Part model, mm, in its own coordinate system. A direction names the side the tool comes from. Give positions to 0.01 mm unless a question says otherwise; leave off trailing zeros. Write each loop counter-clockwise with the first axis right and the second up, starting at its lowest first coordinate (ties: lowest second). Pieces come first, ordered by that corner, then holes. Notation, with made-up numbers: (81.25, 53) - (85.25, 53) arc R19 ccw to (85.25, 89) - close; hole circle Ø8 at (11, 40.5). An arc over 180 degrees is marked (long way). Answer as a JSON object with one key per item and string values. Group by question number.
```python
from build123d import *

# Parameters (mm, degrees)
F0_R     = 7.493
F0_R_2   = 5.08
F0_R_3   = 3.429
F1_DEPTH = 67.4878
F2_R     = 5.08
F2_R_2   = 3.429
F3_DEPTH = 5.08
F4_SIZE  = 1.65099
F5_R     = 3.429
F6_DEPTH = 7.62


# Not quite as in the source:
# - a fillet or chamfer is up to 0.001 mm smaller than in the source, because OpenCascade refuses the exact size


with BuildPart() as f1:
    # F0 (on Top) → F1 (new body)
    with BuildSketch(Plane.XY):
        Circle(F0_R)
        Circle(F0_R_2, mode=Mode.SUBTRACT)
        Circle(F0_R_2)
        Circle(F0_R_3, mode=Mode.SUBTRACT)
    extrude(amount=F1_DEPTH)

    # F2 (on face) → F3 (cut)
    with BuildSketch(Plane(origin=(0, 0, 0), x_dir=(1, 0, 0), z_dir=(0, 0, -1))):
        Circle(F2_R)
        Circle(F2_R_2, mode=Mode.SUBTRACT)
    extrude(amount=-F3_DEPTH, mode=Mode.SUBTRACT)

    # F4 (size 1.651 in the source; OpenCascade refuses exactly that, so slightly less here)
    f4_edges = [f1.edges().sort_by_distance(p)[0] for p in [
        (-3.429, 0, 5.08),
    ]]
    chamfer(f4_edges, length=F4_SIZE)

    # F5 (on face) → F6 (cut)
    with BuildSketch(Plane.XY.offset(67.4878)):
        Polygon((6.6034672536, -0.0838822432), (3.3743777803, 5.6768292731), (-3.2290894733, 5.7607115163), (-6.6034672536, 0.0838822432), (-3.3743777803, -5.6768292731), (3.2290894733, -5.7607115163), align=None)
        Circle(F5_R, mode=Mode.SUBTRACT)
        Circle(F5_R)
    extrude(amount=-F6_DEPTH, mode=Mode.SUBTRACT)


solid = f1.part
```
1) Which spindle directions (+Z, -Z, +X, -X, +Y, -Y) get a long thin tool onto all of the face, cutting with end or side? Do faces 5 (the cylindrical face through (-0.74, -3.35, 32.93)), 6 (the cylindrical face through (-0.661, -5.037, 2.504)), 7 (the flat face through (-4.893, 2.962, 63.731)). Say none if no direction does.
2) Saw through at B-B (z = 30.5). List the corners of the cut face in (x, y).
3) Drop flat-ended pins along their axis: P1, Ø5, axis at x = 0, y = -0.5, coming from the -Z side; P2, Ø6, axis at y = 4, z = 32, coming from the -X side; P3, Ø5, axis at y = 3, z = 60.5, coming from the +X side; P4, Ø8, axis at y = -5, z = 60.5, coming from the +X side. Give the stop position or say it passes through.
4) Two-plate mould, pull along X, no slides. Class faces 1 (the flat face through (5, -2, 0)), 2 (the cylindrical face through (-0.98, 7.43, 33.27)), 3 (the flat face through (5.01, 2.76, 63.73)), 4 (the flat face through (3, 3, 59.868)): +X half, -X half, draft (parallel to the pull), parting line (faces both ways), or undercut.
5) Drill centre lines: line 1 along Y through (x, z) = (0, 3.8); line 2 along Y through (x, z) = (0, 42.5); line 3 along X through (y, z) = (-5.5, 41.5). Where is each one in solid material? Low to high. Write a range as from..to.
Checks:
{
 "1": {"face 5": "+Z, -Z", "face 6": "-Z", "face 7": "+Z"},
 "2": {"outline": "circle Ø14.99 at (0, 0); hole circle Ø6.86 at (0, 0)"},
 "3": {"P1": "through", "P2": "x = -7.43", "P3": "x = 7.48", "P4": "x = 7.43"},
 "4": {"face 1": "draft", "face 2": "parting line", "face 3": "undercut", "face 4": "undercut"},
 "5": {"line 1": "-7.49..-5.08, 5.08..7.49", "line 2": "-7.49..-3.43, 3.43..7.49", "line 3": "-5.09..5.09"}
}
